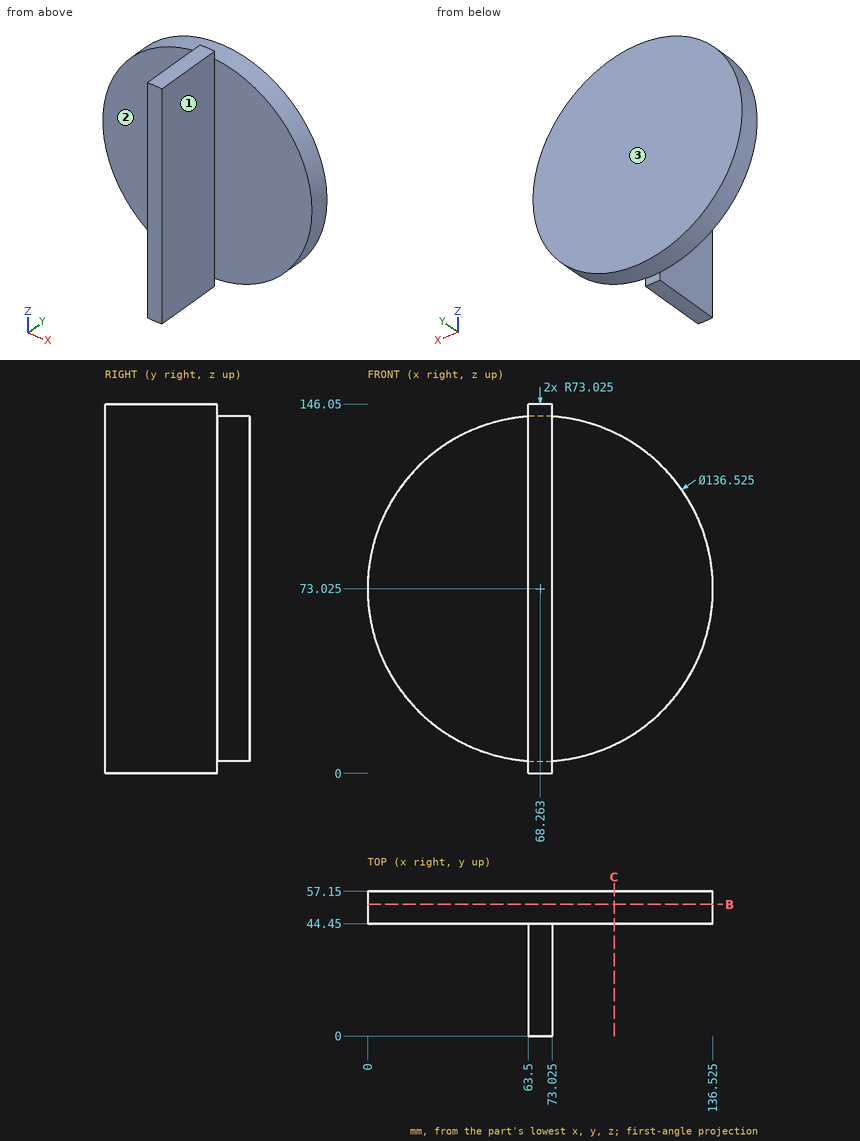
Geometry check sheet. Reference: drawing and pictorial views, mm from the part's lowest x, y, z. A direction names the side the tool comes from. Round coordinates to 2 decimals unless told otherwise and drop trailing zeros. Order: outer loops, then holes, each group sorted by start corner. A loop starts at its lowest first (then second) coordinate and runs counter-clockwise, first axis right, second up.
Q1. Cross-section at C-C, the plane x = 97.5. Enter the section's corners in (y, z), plus the area to 3 significant figures.
Filled sheet:
outline: (44.45, 11.34) - (57.15, 11.34) - (57.15, 134.71) - (44.45, 134.71) - close
area: 1,570 mm2
Q2. Set-up check for the marked faces 1, 2 and 3: record each of +Z, -Z, +X, -X, +Y, -Y from which the full face is reachable in a straight line by a thin tool's end or side.
Filled sheet:
face 1: +Z, -Z, +X, -Y
face 2: +Z, -Z, -X, -Y
face 3: +Z, -Z, +X, -X, +Y
Q3. Scan lines: L1, parallel to X at y = 26, z = 13 (1 decimal); L2, parallel to Y at x = 13, z = 56.5; L3, parallel to Z at x = 67, y = 8.5. Record each from-to range of solid material in increasing order.
Filled sheet:
L1: x = 63.5 to 73
L2: y = 44.45 to 57.15
L3: z = 0.01 to 146.04
Q4. Cross-section at B-B, the plane y = 52. Enter the section's corners in (x, z) (1 decimal).
Filled sheet:
outline: circle Ø136.5 at (68.3, 73)
Q5. Depth check by flat-ended pin: P1, Ø6, axis at y = 43.5, z = 24.5, coming from the +X side; P2, Ø1.5, axis at y = 13, z = 91, coming from the +X side (1 decimal); P3, Ø12, axis at y = 27.5, z = 61.5, coming from the -X side. Enter the tip coordinate at first touch or a pass-through.
Filled sheet:
P1: stops at x = 118.99
P2: stops at x = 73
P3: stops at x = 63.5
